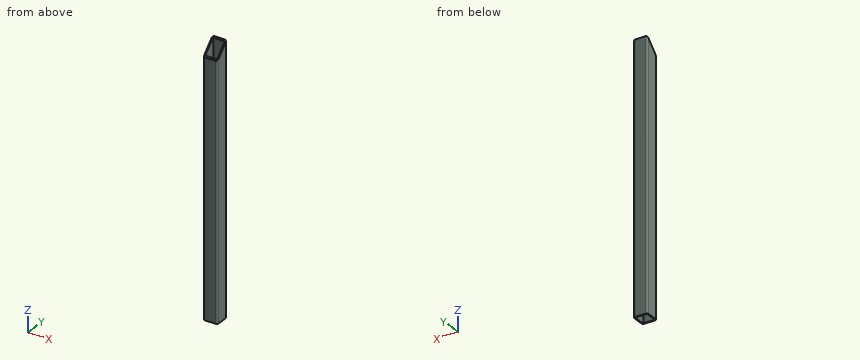
Autodesk Inventor part; units mm, degrees
ref_plane "Start plane" through (0, 0, 30) normal (0, 0, 1) x (1, 0, 0)
ref_plane "End plane" through (0, 0, 600) normal (0, 0, 1) x (1, 0, 0)
ref_plane "Work Plane4" through (425, -558.75, 30) normal (0, 0, -1) x (-1, 0, 0)
ref_plane "Start plane" through (0, 0, 30) normal (0, 0, 1) x (1, 0, 0)
ref_plane "End plane" through (0, 0, 600) normal (0, 0, 1) x (1, 0, 0)
sketch "Sketch" plane through (0, 0, 0) normal (0, 0, 1) x (1, 0, 0)
  line L0 (-15, -11.25) -> (-15, 11.25)
  line L1 (-11.25, 15) -> (11.25, 15)
  line L2 (15, 11.25) -> (15, -11.25)
  line L3 (11.25, -15) -> (-11.25, -15)
  arc A0 (-15, -11.25) -> (-11.25, -15) centre (-11.25, -11.25) ccw
  arc A1 (-11.25, 15) -> (-15, 11.25) centre (-11.25, 11.25) ccw
  arc A2 (15, 11.25) -> (11.25, 15) centre (11.25, 11.25) ccw
  arc A3 (11.25, -15) -> (15, -11.25) centre (11.25, -11.25) ccw
  arc A4 (-11.25, 12.5) -> (-12.5, 11.25) centre (-11.25, 11.25) ccw
  line L4 (-11.25, 12.5) -> (11.25, 12.5)
  arc A5 (12.5, 11.25) -> (11.25, 12.5) centre (11.25, 11.25) ccw
  line L5 (12.5, 11.25) -> (12.5, -11.25)
  arc A6 (11.25, -12.5) -> (12.5, -11.25) centre (11.25, -11.25) ccw
  line L6 (11.25, -12.5) -> (-11.25, -12.5)
  arc A7 (-12.5, -11.25) -> (-11.25, -12.5) centre (-11.25, -11.25) ccw
  line L7 (-12.5, -11.25) -> (-12.5, 11.25)
  line L8 (0, 22.0873) -> (0, -22.0873) construction
  line L9 (-22.0873, 0) -> (22.0873, 0) construction
  dimension "d7" = 3.75
  dimension "d10" = 30
  dimension "d11" = 30
  dimension "d12" = 2.5
  dimension "d15" = 15
  dimension "d16" = 15
extrude "Body" add sketch "Sketch" along normal up to surface (570 mm away) from surface at 30
sketch "Sketch3" plane through (0, 0, 0) normal (0, 0, 1) x (1, 0, 0)
  line L0 (0, 0) -> (10, 0)
ref_plane "Work Plane3" through (0, 0, 0) normal (0, -1, 0) x (1, 0, 0)
sketch "Sketch4" plane through (0, 0, 0) normal (0, -1, 0) x (1, 0, 0)
  line L0 (-2, 30) -> (12, 30)
  line L1 (-2, 600) -> (12, 600)
  dimension "d18" = 570
ref_plane "Work Plane4" through (425, -558.75, 30) normal (0, 0, -1) x (-1, 0, 0)
split "Split1" plane through (425, -558.75, 30) removes the side toward (0, 0, -1)
ref_plane "Work Plane5" through (0, 15, 600) normal (0, -0.7071, 0.7071) x (1, 0, 0)
split "Split2" plane through (0, 15, 600) removes the side toward (0, -0.7071, 0.7071)
ref_plane "Work Plane6" through (385, 11.25, 30) normal (0, 0, -1) x (-1, 0, 0)
split "Split3" plane through (385, 11.25, 30) removes the side toward (0, 0, -1)
equation "\"d7\" = G_IR"
equation "\"d10\" = G_H"
equation "\"d11\" = G_W"
equation "\"d12\" = G_T"
equation "\"d15\" = 0.5 * d10"
equation "\"d16\" = 0.5 * d11"
equation "\"d3\" = G_L"
equation "\"G_W\" = 30"
equation "\"G_H\" = 30"
equation "\"G_T\" = 2.5"
equation "\"G_IR\" = 3.75"
equation "\"G_L\" = d18"
equation "\"G_OFFSET_END\" = 0"
properties part number "DIN EN 10305-5 - 30 x 30 x 2,5  - 570" material "Steel, Mild"
Read the model definition and answer for the solid it produces. Units are mm, in the model's axes. Round coordinates to 2 decimals unless told otherwise and drop trailing zeros. Write each loop counter-clockwise with the first axis right and the second up, starting at its lowest first coordinate (ties: lowest second). Pieces come first, ordered by that corner, then holes. Notation, with made-up numbers: (-1.5, 63) - (37.5, 63) arc R19 cw to (37.5, 76) - close; hole circle Ø4 at (7, 73.5). An arc over 180 degrees is marked (long way). One line per question, with ' | ' between items. Start each with the question number.
1. Find the intervals of material crossed by probe 1 along Y at (x, z) = (-1.5, 510); probe 2 along Z at (x, y) = (13.75, 2), in increasing order. Write a range as [from, to].
2. Section A-A (y = 1) is taken. Determine the outline of the cut face in (x, z).
3. Section B-B (x = -2.5) is taken. Determine the outline of the cut face in (y, z).
4. Section C-C (z = 454) is taken. Determine the outline of the cut face in (x, y), and give its area (3 significant figures).
Filled in:
1) probe 1: [-15, -12.5], [12.5, 15] | probe 2: [30, 587]
2) outline: (-15, 30) - (-12.5, 30) - (-12.5, 586) - (-15, 586) - close; (12.5, 30) - (15, 30) - (15, 586) - (12.5, 586) - close
3) outline: (-15, 30) - (-12.5, 30) - (-12.5, 572.5) - (-15, 570) - close; (12.5, 30) - (15, 30) - (15, 600) - (12.5, 597.5) - close
4) outline: (-15, -11.25) arc R3.75 ccw to (-11.25, -15) - (11.25, -15) arc R3.75 ccw to (15, -11.25) - (15, 11.25) arc R3.75 ccw to (11.25, 15) - (-11.25, 15) arc R3.75 ccw to (-15, 11.25) - close; hole (-12.5, -11.25) arc R1.25 ccw to (-11.25, -12.5) - (11.25, -12.5) arc R1.25 ccw to (12.5, -11.25) - (12.5, 11.25) arc R1.25 ccw to (11.25, 12.5) - (-11.25, 12.5) arc R1.25 ccw to (-12.5, 11.25) - close | area: 264 mm²
